```python
from build123d import *

# Parameters (mm, degrees)
F1_DEPTH       = 20
F4_REACH       = 59.8904911491
F6_REACH       = 49.0077165035
F8_DEPTH       = 17.7213446758
F8_DEPTH_BACK  = 25
F10_REACH      = 31.5666498146
F12_DEPTH      = 19.1713446758
F12_DEPTH_BACK = 31.9213446758
F13_R          = 2.5
F14_DEPTH      = 5


with BuildPart() as f1:
    # F0 (on Top) → F1 (new body)
    with BuildSketch(Plane.XY):
        Polygon((7.7645713531, -28.9777747887), (0, 0), (7.7645713531, 28.9777747887), (-13.4857968253, 34.6717937809), (-22.776075969, 0), (-13.4857968253, -34.6717937809), align=None)
    extrude(amount=F1_DEPTH)

    f4_end = Plane(origin=(0, 0, 20), x_dir=(0, 0, 1), z_dir=(0, 1, 0))
    # F3 (on face) → F4 (cut, up to a plane its end follows)
    with BuildSketch(Plane(origin=(7.7645713531, -28.9777747887, 0), x_dir=(0.9659258263, 0.2588190451, 0), z_dir=(0.2588190451, -0.9659258263, 0))):
        Polygon((-13.3987803669, 15), (-17.1487803669, 8.5048094716), (-4.8512196331, 1.4048094716), (-1.1012196331, 7.9), (0, 7.9), (0, 20), (-13.3987803669, 20), align=None)
    f4_long = extrude(amount=-F4_REACH, mode=Mode.PRIVATE)
    add(split(f4_long, bisect_by=f4_end, keep=Keep.BOTTOM, mode=Mode.PRIVATE), mode=Mode.SUBTRACT)

    f6_end = Plane(origin=(0, 0, 20), x_dir=(0, 0, 1), z_dir=(0, 1, 0))
    # F5 (on face) → F6 (cut, up to a plane its end follows)
    with BuildSketch(Plane(origin=(7.7645713531, -28.9777747887, 0), x_dir=(0.9659258263, 0.2588190451, 0), z_dir=(0.2588190451, -0.9659258263, 0))):
        Polygon((-22, 20), (-22, 10.1022505884), (-17.7289073858, 17.5), (-13.3987803669, 15), (-13.3987803669, 20), align=None)
    f6_long = extrude(amount=-F6_REACH, mode=Mode.PRIVATE)
    add(split(f6_long, bisect_by=f6_end, keep=Keep.BOTTOM, mode=Mode.PRIVATE), mode=Mode.SUBTRACT)

    # F7 (on face) → F8 (cut, two sides)
    with BuildSketch(Plane(origin=(-15.9805432759, -4.2819736654, 9.5518420887), x_dir=(-0.1923952931, 0.9745560663, 0.1149979338), z_dir=(0.8365163037, 0.224143868, -0.5))) as f8_sk:
        Polygon((-28.8989639862, 10.218925907), (-36.8281195036, 11.2812313158), (-37.8240308243, 3.8476480182), (-29.8948753069, 2.7853426095), align=None)
    extrude(amount=-F8_DEPTH, mode=Mode.SUBTRACT)
    extrude(f8_sk.sketch, amount=F8_DEPTH_BACK, mode=Mode.SUBTRACT)

    f10_end = Plane(origin=(0, 0, 20), x_dir=(0, 0, 1), z_dir=(0, 1, 0))
    # F9 (on face) → F10 (cut, up to a plane its end follows)
    with BuildSketch(Plane(origin=(7.7645713531, -28.9777747887, 0), x_dir=(0.9659258263, 0.2588190451, 0), z_dir=(0.2588190451, -0.9659258263, 0))):
        Polygon((0, 7.9), (-1.1012196331, 7.9), (0, 7.2642105484), align=None)
    f10_long = extrude(amount=-F10_REACH, mode=Mode.PRIVATE)
    add(split(f10_long, bisect_by=f10_end, keep=Keep.BOTTOM, mode=Mode.PRIVATE), mode=Mode.SUBTRACT)

    # F11 (on face) → F12 (cut, two sides)
    with BuildSketch(Plane(origin=(-4.1020117628, -1.0991307392, 2.4518420887), x_dir=(0.1923952931, -0.9745560663, -0.1149979338), z_dir=(-0.8365163037, -0.224143868, 0.5))) as f12_sk:
        Polygon((8.7836172997, 7.5239804569), (-1.127827097, 6.196098696), (-0.1319157763, -1.2374846015), (9.7795286204, 0.0903971594), align=None)
    extrude(amount=-F12_DEPTH, mode=Mode.SUBTRACT)
    extrude(f12_sk.sketch, amount=F12_DEPTH_BACK, mode=Mode.SUBTRACT)

    # F13 (on face) → F14 (cut, through all)
    with BuildSketch(Plane(origin=(-20.1631247946, -5.4026930056, 12.0518420887), x_dir=(0.1923952931, -0.9745560663, -0.1149979338), z_dir=(-0.8365163037, -0.224143868, 0.5))):
        with Locations((19.4084412411, 4.6381834861)):
            Circle(F13_R)
    extrude(amount=-F14_DEPTH, mode=Mode.SUBTRACT)

    # F15: F1 across plane


with BuildPart() as f1_1:
    add(f1.part)
    add(f1.part.mirror(Plane.XZ), mode=Mode.INTERSECT)


solid = f1_1.part
```
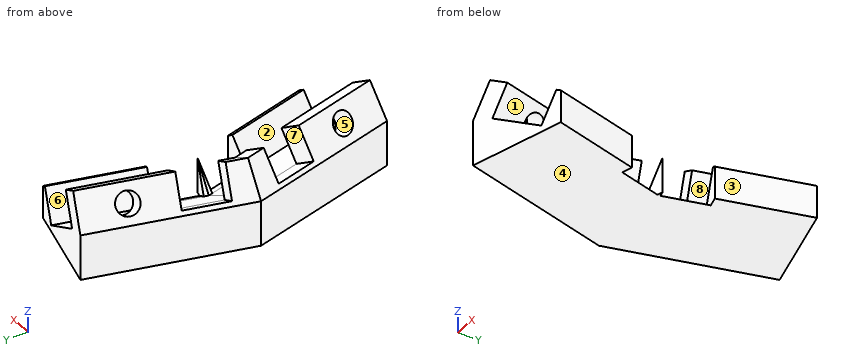
Geometry: final body of the model. Coordinates: model frame, mm. Face numbers are marked on the shaded views. A direction names the side the tool comes from. Coordinates: 2 decimals unless noted, no trailing zeros. Write each loop counter-clockwise with the first axis right and the second up, starting at its lowest first coordinate (ties: lowest second). Pieces come first, ordered by that corner, then holes. Notation, with made-up numbers: M 39.5,17 L 45.5,17 A15 cw 45.5,31 Z; hole C 36,58.5 d9. An arc over 180 degrees is marked long. Use CSV: the item, a comma, the result in double quotes. Start each with the question number.
1. Ray query, probe 1 along X at (y, z) = (-27.5, 7); probe 2 along X at (y, z) = (-16, 7.75); probe 3 along X at (y, z) = (-25.5, 12.5). Return the intervals inside material, ascending.
2. Cut plane C-C on x = -6. Return the cut outline in (y, z), plus the area to 3 significant figures.
3. Reachability of the marked faces 1, 2, 3, 4 and 5 from +Z, -Z, +X, -X, +Y, -Y: full face, straight path, thin tool, end or side. Return the list, or none.
4. First-contact query: P1, Ø6, axis at y = 4, z = 9, coming from the -X side; P2, Ø4, axis at x = -16, y = -7, coming from the -Z side; P3, Ø4, axis at y = 13.5, z = 12, coming from the +X side; P4, Ø4, axis at x = -6, z = 2, coming from the -Y side. Flat tips, straight axial feed; report the tip coordinate or a pass-through.
5. Cut plane A-A on z = 3.5. Return the cut outline in (x, y), plus the area to 3 significant figures.
6. Cut plane D-D on y = -7. Return the cut outline in (x, z).
7. Cut plane B-B on z = 16.75. Return the cut outline in (x, y), plus the area to 3 significant figures.
8. Mould query, pull axis Z, two halves, no side actions, for the marked faces 6, 7 and 8. Classes: pulls with the +Z half, pulls with the -Z half, needs draft (parallel to the pull), parting line crosses it, or undercut.
Entries:
1,probe 1,"-15.41 to -7.69, 5.69 to 7.37"
1,probe 2,"-18.49 to -12.11, 3.06 to 3.42"
1,probe 3,"-9.49 to -8.53"
2,outline,"M -32.67,0 L 32.67,0 L 32.67,6.83 L 0,1.95 L -32.67,6.83 Z; M -32.67,13.53 L -29.38,15 L -32.67,15.49 Z; M 29.38,15 L 32.67,13.53 L 32.67,15.49 Z"
2,area,"293 mm²"
3,face 1,"+X"
3,face 2,"+Z"
3,face 3,"+Z, -Z, +X"
3,face 4,"-Z, +X, -X, +Y, -Y"
3,face 5,"none"
4,P1,"x = -22.51"
4,P2,"z = 0"
4,P3,"x = -10.74"
4,P4,"y = -33.2"
5,outline,"M -22.78,0 L -13.49,-34.67 L -0.43,-31.17 L -8.78,0 L -0.43,31.17 L -13.49,34.67 Z; M -3.77,0 L -3.59,-0.66 L -1.14,0 L -3.59,0.66 Z; M -1.01,-10.32 L 4.25,-29.92 L 7.76,-28.98 L 2.51,-9.37 Z; M -1.01,10.32 L 2.51,9.37 L 7.76,28.98 L 4.25,29.92 Z"
5,area,"1,070 mm²"
6,outline,"M -20.9,0 L -0.63,0 L -20.36,11 L -20.9,10.1 Z"
7,outline,"M -18.8,0 L -17.62,-4.42 L -15.95,-3.97 L -17.01,0 L -15.95,3.97 L -17.62,4.42 Z; M -15.03,-14.07 L -9.78,-33.68 L -8.11,-33.23 L -13.36,-13.63 Z; M -15.03,14.07 L -13.36,13.63 L -8.11,33.23 L -9.78,33.68 Z"
7,area,"85.3 mm²"
8,face 6,"pulls with the +Z half"
8,face 7,"needs draft"
8,face 8,"undercut"
